Source: CAD feature listing. Evaluate the final solid. Frame: model axes, mm. Coordinates: 2 decimals unless noted, no trailing zeros.
Autodesk Fusion 360 part; units mm, degrees
sketch "Sketch2" plane through (0, 0, 0) normal (0, 0, 1) x (1, 0, 0)
  line L0 (-214.5, -61) -> (-214.5, 61)
  line L1 (-214.5, -61) -> (214.5, 61) construction
  line L2 (-214.5, 61) -> (214.5, 61)
  circle A0 centre (42.5, -3.3) radius 4.1
  line L3 (214.5, -61) -> (-214.5, 61) construction
  line L4 (214.5, 61) -> (214.5, -61)
  line L5 (214.5, -61) -> (-214.5, -61)
  line L6 (-214.5, 0) -> (214.5, 0) construction
  line L7 (-214.5, -3.3) -> (214.5, -3.3) construction
  line L8 (42.5, 61) -> (42.5, -61) construction
  circle A1 centre (42.5, 51) radius 2.1
  line L9 (-214.5, 51) -> (214.5, 51) construction
  circle A2 centre (42.5, -3.3) radius 22.5 construction
  circle A3 centre (42.5, 19.2) radius 2.1
  circle A4 centre (23.0144, 7.95) radius 2.1
  circle A5 centre (23.0144, -14.55) radius 2.1
  circle A6 centre (42.5, -25.8) radius 2.1
  circle A7 centre (61.9856, -14.55) radius 2.1
  circle A8 centre (61.9856, 7.95) radius 2.1
  line L10 (-194.5, 61) -> (-194.5, -61) construction
  line L11 (194.5, 61) -> (194.5, -61) construction
  circle A9 centre (-167.5, 51) radius 2.1
  circle A10 centre (-97.5, 51) radius 2.1
  circle A11 centre (-27.5, 51) radius 2.1
  circle A12 centre (112.5, 51) radius 2.1
  circle A13 centre (182.5, 51) radius 2.1
  circle A14 centre (112.5, -51) radius 2.1
  line L12 (-214.5, -51) -> (214.5, -51) construction
  circle A15 centre (-27.5, -51) radius 2.1
  circle A16 centre (-167.5, -51) radius 2.1
  circle A17 centre (182.5, -51) radius 2.1
  circle A18 centre (-97.5, -51) radius 2.1
  circle A19 centre (42.5, -51) radius 2.1
  circle A20 centre (-204.5, 0) radius 2.1
  circle A21 centre (204.5, 0) radius 2.1
  dimension "d11" = 122
  dimension "d12" = 429
  dimension "d14" = 8.2
  dimension "d18" = 3.3
  dimension "d20" = 172
  dimension "d21" = 4.2
  dimension "d23" = 10
  dimension "d24" = 45
  dimension "d25" = 4.2
  dimension "d27" = 360
  dimension "d30" = 70
  dimension "d31" = 0
  dimension "d32" = 20
  dimension "d33" = 20
  dimension "d34" = 4.2
  dimension "d35" = 10
  dimension "d36" = 4.2
  dimension "d37" = 10
extrude "Extrude2" add sketch "Sketch2" along normal blind 3.5
sketch "Sketch3" plane through (0, 0, 3.5) normal (0, 0, 1) x (-1, 0, 0)
  circle A0 centre (-42.5, 3.3) radius 4
  line L0 (-214.5, 61) -> (-214.5, -61)
  line L1 (-214.5, -61) -> (214.5, -61)
  line L2 (214.5, -61) -> (214.5, 61)
  line L3 (214.5, 61) -> (-214.5, 61)
  line L4 (-130, -50) -> (-141.5967, -50) construction
  line L5 (-141.5967, -50) -> (-141.5967, -60) construction
  line L6 (-141.5967, -60) -> (-130, -60) construction
  line L7 (-130, -60) -> (-130, -50) construction
  circle A1 centre (-182.5, 51) radius 2.1
  circle A2 centre (97.5, 51) radius 2.1
  circle A3 centre (-42.5, 51) radius 2.1
  circle A4 centre (204.5, 0) radius 2.1
  circle A5 centre (-204.5, 0) radius 2.1
  circle A6 centre (167.5, 51) radius 2.1
  circle A7 centre (97.5, -51) radius 2.1
  circle A8 centre (27.5, -51) radius 2.1
  circle A9 centre (-112.5, -51) radius 2.1
  circle A10 centre (-182.5, -51) radius 2.1
  circle A11 centre (-112.5, 51) radius 2.1
  circle A12 centre (27.5, 51) radius 2.1
  circle A13 centre (167.5, -51) radius 2.1
  circle A14 centre (-61.9856, -7.95) radius 2.1
  circle A15 centre (-61.9856, 14.55) radius 2.1
  circle A16 centre (-42.5, 25.8) radius 2.1
  circle A17 centre (-23.0144, 14.55) radius 2.1
  circle A18 centre (-23.0144, -7.95) radius 2.1
  circle A19 centre (-42.5, -19.2) radius 2.1
  circle A20 centre (-42.5, -51) radius 2.1
  circle A21 centre (-42.5, 3.3) radius 4.1
  line L8 (-214.5, 61) -> (-214.5, -61)
  line L9 (-214.5, -61) -> (214.5, -61)
  line L10 (214.5, -61) -> (214.5, 61)
  line L11 (214.5, 61) -> (-214.5, 61)
Q1. Pin query (flat end, axial travel): P1, Ø7.5, axis at x = 42.5, y = -3.3, coming from the -Z side. Return the tip coordinate at first contact, or that it passes through.
Solutions:
P1: passes through
Q2. Material intervals for line 1 along Y through (x, z) = (-167.5, 2.45); line 2 along X through (y, z) = (-3, 2.25), sorted ascending.
Solutions:
line 1: y = -61 to -53.1, -48.9 to 48.9, 53.1 to 61
line 2: x = -214.5 to 38.41, 46.59 to 214.5
Q3. Pull-direction query (X, two-part tool) for faces 1 (the cylindrical face through (38.404, -3.48, 1.726)), 2 (the flat face through (-3, 1, 3.5)); classes: pulls with the +X half, pulls with the -X half, needs draft (parallel to the pull), parting line crosses it, or undercut.
Solutions:
face 1: undercut
face 2: needs draft
